Source: three-view drawing plus pictorial views. Frame: mm from the lowest corner of the part. Coordinates: 2 decimals unless noted, no trailing zeros. Order: outer loops, then holes, each group sorted by start corner. A loop starts at its lowest first (then second) coordinate and runs counter-clockwise, first axis right, second up. Notation, with made-up numbers: (13.25, 3.5) - (17.25, 3.5) arc R21 ccw to (17.25, 38.5) - close; hole circle Ø4 at (75, 17.25). An arc over 180 degrees is marked (long way). One line per question, with ' | ' between items.
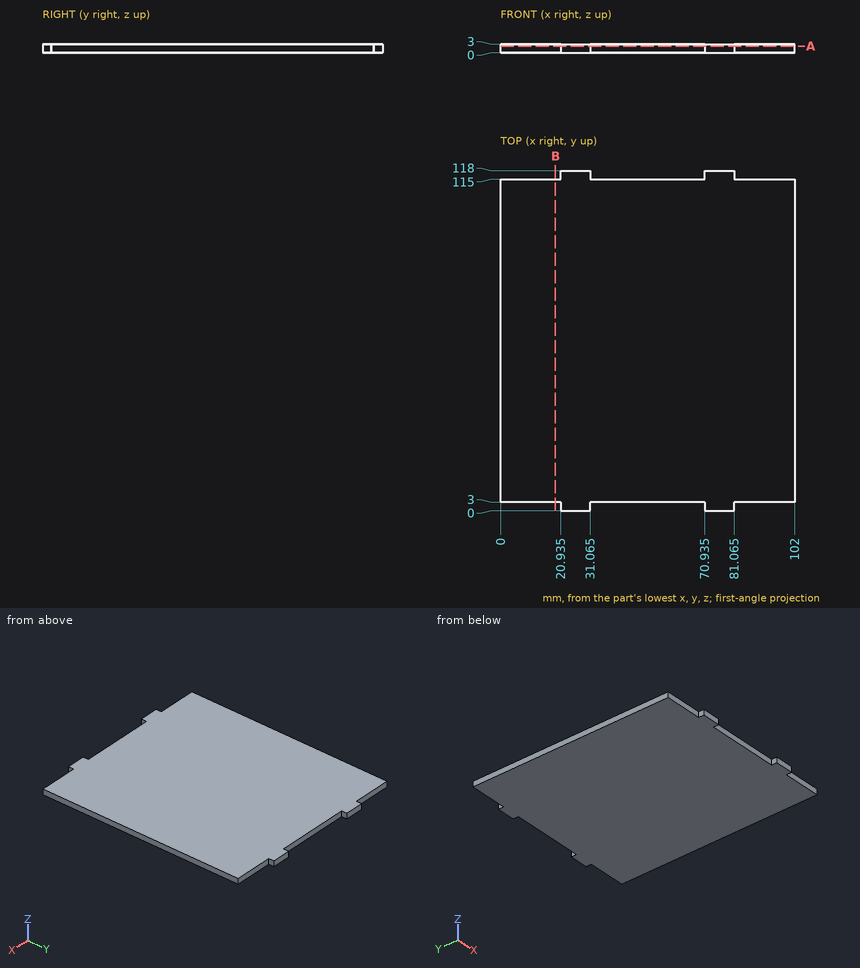
(1) Cut plane A-A (z = 2.25). Return the cut outline in (x, y) (3 decimals).
Taken from the geometry:
outline: (0, 3) - (20.935, 3) - (20.935, 0) - (31.065, 0) - (31.065, 3) - (70.935, 3) - (70.935, 0) - (81.065, 0) - (81.065, 3) - (102, 3) - (102, 115) - (81.065, 115) - (81.065, 118) - (70.935, 118) - (70.935, 115) - (31.065, 115) - (31.065, 118) - (20.935, 118) - (20.935, 115) - (0, 115) - close
(2) Cut plane B-B (x = 19). Return the cut outline in (y, z).
Taken from the geometry:
outline: (3, 0) - (115, 0) - (115, 3) - (3, 3) - close
(3) Material intervals for L1, parallel to Y at x = 68, z = 0.6, sorted ascending. Write a range as from..to.
Taken from the geometry:
L1: y = 3..115
(4) Pin query (flat end, axial travel): P1, Ø1.5, axis at y = 2, z = 1, coming from the +X side (3 decimals); P2, Ø1.5, axis at x = 46, z = 0.5, coming from the -Y side; P3, Ø1.5, axis at x = 60, z = 2, coming from the +Y side; P4, Ø1, axis at x = 29, z = 1, coming from the -Y side. Return the tip coordinate at first contact, or that it passes through.
Taken from the geometry:
P1: stops at x = 81.065 | P2: stops at y = 3 | P3: stops at y = 115 | P4: stops at y = 0
